Solid Edge part; units mm, degrees
sketch "Sketch1" plane through (0, 0, 0) normal (0, 0, 1) x (1, 0, 0)
  circle A0 centre (-62.269, 22.0507) radius 250
  circle A1 centre (-62.269, 22.0507) radius 75
extrude "Protrusion1" add sketch "Sketch1" along normal blind 50
sketch "Sketch2" plane through (-62.269, 22.0507, 50) normal (0, 0, 1) x (0, 1, 0)
  arc A0 (150, 0) -> (26.0472, 147.7212) centre (0, 0) ccw
  line L0 (26.0472, 147.7212) -> (52.0945, 295.4423)
  line L1 (52.0945, 295.4423) -> (379.3774, 186.8257)
  line L2 (379.3774, 186.8257) -> (365.0673, 0)
  line L3 (150, 0) -> (365.0673, 0)
extrude "Cutout1" cut sketch "Sketch2" against normal through all
sketch "Sketch3" plane through (-69.8074, 22.0507, 50) normal (0, 0, 1) x (0, 1, 0)
  line L0 (43.412, 238.6635) -> (-252.0303, 186.5691)
  line L1 (-252.0303, 186.5691) -> (-35.9633, 306.8202)
  line L2 (-35.9633, 306.8202) -> (43.412, 238.6635)
extrude "Cutout2" cut sketch "Sketch3" against normal through all
sketch "Sketch4" plane through (-77.1168, 29.5891, 50) normal (0, 0, 1) x (0.9396926, -0.3420201, 0)
  line L0 (-8.4693, 182.9176) -> (41.5307, 182.9176)
  line L1 (41.5307, 182.9176) -> (41.5307, 232.9176)
  line L2 (41.5307, 232.9176) -> (-8.4693, 232.9176)
  line L3 (-8.4693, 232.9176) -> (-8.4693, 182.9176)
extrude "Cutout3" cut sketch "Sketch4" against normal through all
pattern_circular "Pattern1" count 3 over 360 about axis through (-62.269, 22.0507, 50) along (0, 0, -1) of "Cutout1", "Cutout3", "Cutout2"
Can you work these out from the model? Positions are in its coordinate system, mm. A direction names the side the tool comes from. Coordinates: 2 decimals unless noted, no trailing zeros. Write each loop counter-clockwise with the first axis right and the second up, starting at its lowest first coordinate (ties: lowest second). Pieces come first, ordered by that corner, then holes. Notation, with made-up numbers: (23.25, 72.25) -> (29.25, 72.25) arc R7 ccw to (29.25, 78.25) -> close; hole circle Ø9 at (39.5, 32). An arc over 180 degrees is marked (long way). Write each question's results on one line, items separated by ' | '. Start each with the question number.
Q1. Imagine slicing it at B-B (x = -53.5). Write out the boundary of the cut face in (y, z).
Q2. Imagine slicing it at C-C (z = 38). Write out the boundary of the cut face in (x, y), then the cut area to 3 significant figures.
Q3. Imagine slicing it at D-D (x = -225.5). Write out the boundary of the cut face in (y, z).
Q4. If I drill on probe 1 along Y at (x, z) = (66, 47); probe 2 along Y at (x, z) = (52.5, 44); probe 3 along X at (y, z) = (89, 28.5), over which ranges is the centre line in solid material (lowest first)?
Q5. I'm going to push flat-ended pins straight in: pin 1 (12 mm diameter, centred on x = -237, z = 11.5, fed in from -Y); pin 2 (5 mm diameter, centred on y = 184.5, z = 20.5, fed in from +X); pin 3 (5 mm diameter, centred on x = -260, z = 13.5, fed in from +Y). Where does each tip first touch, or does it pass through?
Q6. Imagine slicing it at A-A (y = 35). Write out the boundary of the cut face in (x, z), then the cut area to 3 significant figures.
Q7. We'd pull the mould along X, two halves only. Please class faces 1 (the face through (130.7, -122.7, 25.4)), 2 (the face through (-234.87, -77.6, 25.35)), 3 (the face through (-284.102, -72.739, 25.35)): +X half, -X half, draft (parallel to the pull), parting line (faces both ways), or undercut.
Q8. On a 3-axis mill with a long thin cutter (end or side, diameter ignored), from which of +Z, -Z, +X, -X, +Y, -Y can I reach the whole of each face in a straight line? I mean faces 4 (the face through (-273, 10.28, 25.35)), 5 (the face through (32.9, 210.43, 25.35)), 6 (the face through (-62.269, 221, 25)), 7 (the face through (92.043, -122.958, 25.35)). Say none if no direction works.
Taken from the geometry:
1) outline: (-127.69, 0) -> (-52.43, 0) -> (-52.43, 50) -> (-127.69, 50) -> close; (96.54, 0) -> (268.86, 0) -> (268.86, 50) -> (96.54, 50) -> close
2) outline: (-308.47, 65.46) -> (-297.96, 5.88) -> (-248.72, 14.56) -> (-240.04, -34.68) -> (-289.28, -43.36) -> (-278.78, -102.95) -> (-192.17, -52.95) arc R150 ccw to (-10.97, -118.9) -> (23.24, -212.87) -> (69.59, -173.98) -> (37.45, -135.68) -> (75.75, -103.54) -> (107.89, -141.84) -> (154.24, -102.95) -> (67.63, -52.95) arc R150 ccw to (34.15, 136.96) -> (98.43, 213.56) -> (41.57, 234.26) -> (24.47, 187.27) -> (-22.51, 204.37) -> (-5.41, 251.36) -> (-62.27, 272.05) -> (-62.27, 172.05) arc R150 ccw to (-209.99, 48.1) -> close; hole circle Ø150 at (-62.27, 22.05) | area: 82,200 mm^2
3) outline: (-72.19, 0) -> (50.83, 0) -> (50.83, 50) -> (-72.19, 50) -> close
4) probe 1: y = -176.99 to -169.71, -111.72 to 99.81, 174.92 to 225.36 | probe 2: y = -188.32 to -153.62, -123.05 to 118.63, 158.83 to 230.28 | probe 3: x = -196.5 to -96.07, -28.46 to 71.96
5) pin 1: stops at y = -82.29 | pin 2: stops at x = 76.14 | pin 3: stops at y = 57.36
6) outline: (-303.1, 0) -> (-136.14, 0) -> (-136.14, 50) -> (-303.1, 50) -> close; (11.6, 0) -> (87.17, 0) -> (87.17, 50) -> (11.6, 50) -> close | area: 12,100 mm^2
7) face 1: +X half | face 2: undercut | face 3: -X half
8) face 4: +Z, -Z | face 5: +Z, -Z, +Y | face 6: +Z, -Z, -X, +Y | face 7: +Z, -Z, -Y
